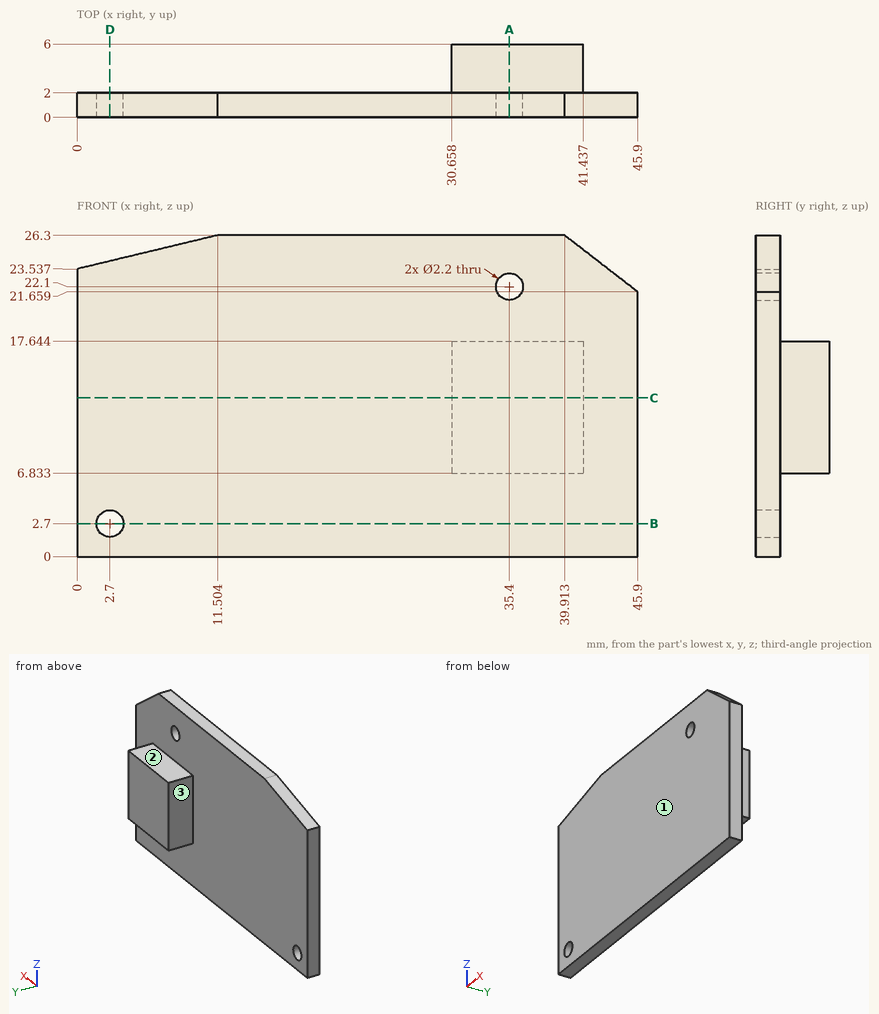
Here's the drawing with two shaded views (mm, measured from the low corner). I have some questions. A direction names the side the tool comes from. Give positions to 0.01 mm unless a question says otherwise; leave off trailing zeros. Loops run counter-clockwise (first coordinate to the right, second up) from the corner with the lowest first, then second, coordinate; pieces in that order, holes last. Notation, with made-up numbers: M -11.75,61.25 L 18.25,61.25 A15 ccw 18.25,80.25 Z; hole C -18.75,10.25 d4. An arc over 180 degrees is marked long. Answer in a Markdown table with one row per item.
1. Suppose I cut it at A-A on x = 35.4. Write out the boundary of the cut face in (y, z).
Taken from the geometry:
| item | result |
|---|---|
| outline | M 0,0 L 2,0 L 2,6.83 L 6,6.83 L 6,17.64 L 2,17.64 L 2,21 L 0,21 Z; M 0,23.2 L 2,23.2 L 2,26.3 L 0,26.3 Z |
2. Which directions (+Z, -Z, +X, -X, +Y, -Y) give clear straight access to the entire face, cutting with the end or side of a thin tool? Please do the marked faces 1, 2 and 3.
Taken from the geometry:
| item | result |
|---|---|
| face 1 | +Z, -Z, +X, -X, -Y |
| face 2 | +Z, +X, -X, +Y |
| face 3 | +Z, -Z, -X, +Y |
3. Suppose I cut it at D-D on x = 2.7. Write out the boundary of the cut face in (y, z) (1 decimal).
Taken from the geometry:
| item | result |
|---|---|
| outline | M 0,0 L 2,0 L 2,1.6 L 0,1.6 Z; M 0,3.8 L 2,3.8 L 2,24.2 L 0,24.2 Z |
4. Suppose I cut it at C-C on z = 13. Write out the boundary of the cut face in (x, y).
Taken from the geometry:
| item | result |
|---|---|
| outline | M 0,0 L 45.9,0 L 45.9,2 L 41.44,2 L 41.44,6 L 30.66,6 L 30.66,2 L 0,2 Z |
5. If I drill on line 1 along Y through (x, z) = (21.5, 3); line 2 along X through (y, z) = (4.3, 8.5); line 3 along Z through (x, y) = (39.5, 5.75), over which ranges is the centre line in solid material (lowest first)?
Taken from the geometry:
| item | result |
|---|---|
| line 1 | y = 0 to 2 |
| line 2 | x = 30.66 to 41.44 |
| line 3 | z = 6.83 to 17.64 |
6. For pin 1 Ø2 at (x, z) = (35.4, 22.1) entering from -Y; pin 2 Ø1.2 at (x, y) = (38.5, 4) entering from +Z; pin 3 Ø1.2 at (y, z) = (3.5, 13) entering from -X; pin 4 Ø1.5 at (y, z) = (2, 23.5) entering from +X, each with a flat end and sliding along its axis, tell me the tip position at first contact or that it passes through.
Taken from the geometry:
| item | result |
|---|---|
| pin 1 | passes through |
| pin 2 | stops at z = 17.64 |
| pin 3 | stops at x = 30.66 |
| pin 4 | stops at x = 44.49 |
7. Suppose I cut it at B-B on z = 2.7. Write out the boundary of the cut face in (x, y).
Taken from the geometry:
| item | result |
|---|---|
| outline | M 0,0 L 1.6,0 L 1.6,2 L 0,2 Z; M 3.8,0 L 45.9,0 L 45.9,2 L 3.8,2 Z |
